from build123d import *

# Parameters (mm, degrees)
SKETCH1_W           = 19
SKETCH1_H           = 35.5
SKETCH1_R           = 1.3
SKETCH1_W_2         = 13
SKETCH1_H_2         = 23.5
BOSS_EXTRUDE1_DEPTH = 4.5


with BuildPart() as part:
    # Sketch1 → Boss-Extrude1 (new body)
    with BuildSketch(Plane(origin=(0, 0, 0), x_dir=(1, 0, 0), z_dir=(0, 1, 0))):
        Rectangle(SKETCH1_W, SKETCH1_H)
        with Locations((0, 13.5)):
            Circle(SKETCH1_R, mode=Mode.SUBTRACT)
        with Locations((0, -13.5)):
            Circle(SKETCH1_R, mode=Mode.SUBTRACT)
        Rectangle(SKETCH1_W_2, SKETCH1_H_2, mode=Mode.SUBTRACT)
    extrude(amount=BOSS_EXTRUDE1_DEPTH)


solid = part.part
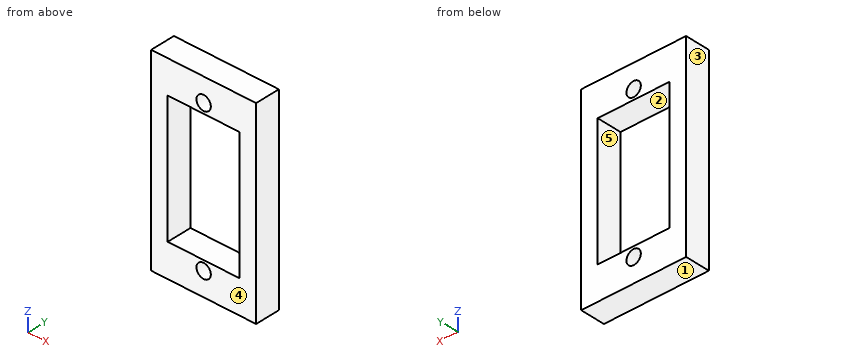
Model file for the job. Use its own axes, mm. Face numbers are marked on the shaded views. A direction names the side the tool comes from. Give positions to 0.01 mm unless a question says otherwise; leave off trailing zeros. Order: outer loops, then holes, each group sorted by start corner. A loop starts at its lowest first (then second) coordinate and runs counter-clockwise, first axis right, second up. Notation, with made-up numbers: (61.25, 47.25) - (72.25, 47.25) arc R19 cw to (72.25, 66.25) - close; hole circle Ø3 at (37.25, 28.5). An arc over 180 degrees is marked (long way). Write item = value, one per line. Start each with the question number.
1. Two-plate mould, pull along X, no slides. Class the marked faces 1, 2 and 3: pulls with the +X half, pulls with the -X half, needs draft (parallel to the pull), parting line crosses it, or undercut.
2. Which spindle directions (+Z, -Z, +X, -X, +Y, -Y) get a long thin tool onto all of the face, cutting with end or side? Do the marked faces 4 and 5. Say none if no direction does.
3. Cut at C-C, the plane y = 4.1. List the corners of the cut face in (x, z), and give its area (3 significant figures).
4. Cut at A-A, the plane x = -1.75. List the corners of the cut face in (y, z), and give its area (3 significant figures).
5. Cut at B-B, the plane z = -10.5. List the corners of the cut face in (x, y).
6. Drop a flat-ended pin along its axis: P1, Ø2, axis at x = 0, z = -13.5, coming from the -Y side. Give the stop position or say it passes through.
7. Probe line 1 along Z through (x, y) = (0, 2.3); line 2 along X through (y, z) = (0.5, 9.5); line 3 along Z through (x, y) = (2.75, 1.1). List the from-to ranges inside material, lowest first.
Taken from the geometry:
q1.face_1 = needs draft
q1.face_2 = undercut
q1.face_3 = pulls with the -X half
q2.face_4 = +Z, -Z, +X, -X, -Y
q2.face_5 = +Y, -Y
q3.outline = (-9.5, -17.75) - (9.5, -17.75) - (9.5, 17.75) - (-9.5, 17.75) - close; hole (-6.5, -11.75) - (6.5, -11.75) - (6.5, 11.75) - (-6.5, 11.75) - close; hole circle Ø2.6 at (0, -13.5); hole circle Ø2.6 at (0, 13.5)
q3.area = 358 mm²
q4.outline = (0, -17.75) - (4.5, -17.75) - (4.5, -11.75) - (0, -11.75) - close; (0, 11.75) - (4.5, 11.75) - (4.5, 17.75) - (0, 17.75) - close
q4.area = 54.0 mm²
q5.outline = (-9.5, 0) - (-6.5, 0) - (-6.5, 4.5) - (-9.5, 4.5) - close; (6.5, 0) - (9.5, 0) - (9.5, 4.5) - (6.5, 4.5) - close
q6.P1 = through
q7.line_1 = -17.75 to -14.8, -12.2 to -11.75, 11.75 to 12.2, 14.8 to 17.75
q7.line_2 = -9.5 to -6.5, 6.5 to 9.5
q7.line_3 = -17.75 to -11.75, 11.75 to 17.75
